Autodesk Inventor part; units mm, degrees
ref_plane "YZ Plane" through (0, 0, 0) normal (1, 0, 0) x (0, 1, 0)
ref_plane "XZ Plane" through (0, 0, 0) normal (0, 1, 0) x (-1, 0, 0)
ref_plane "XY Plane" through (0, 0, 0) normal (0, 0, 1) x (1, 0, 0)
sketch "Boceto1" plane through (0, 0, 0) normal (0, 1, 0) x (-1, 0, 0)
  line L0 (200, 200) -> (-200, 200)
  line L1 (-200, 200) -> (-200, -200)
  line L2 (-200, -200) -> (200, -200)
  line L3 (200, -200) -> (200, 200)
  point P0 (0, 0)
  dimension "d0" = 400
  dimension "L" = 400
  dimension "d2" = 200
  dimension "d3" = 200
extrude "Extrusión1" add sketch "Boceto1" along normal blind 150
sketch "Boceto3" plane through (0, 150, 0) normal (0, 1, 0) x (1, 0, 0)
  circle A0 centre (0, 160) radius 10
  line L0 (200, 200) -> (-200, 200)
  point P0 (0, 0)
  dimension "d6" = 20
  dimension "d9" = 40
extrude "Extrusión2" cut sketch "Boceto3" against normal blind 153.75
ref_plane "Plano de trabajo1" through (0, 0, 200) normal (1, 0, 0) x (0, 0, -1)
ref_plane "Plano de trabajo2" through (-200, 0, 0) normal (0, 0, 1) x (1, 0, 0)
equation "\"d0\" = L"
properties part number "CajaBoya"
Here's how the part is built. I have some questions about the finished solid (model axes, mm). Round coordinates to 2 decimals unless told otherwise and drop trailing zeros. Write each loop counter-clockwise with the first axis right and the second up, starting at its lowest first coordinate (ties: lowest second). Pieces come first, ordered by that corner, then holes.
1. I need wall thicknesses on L1, parallel to X at y = 68.5, z = -160; L2, parallel to Z at x = 0, y = 87.5. Which ranges of each line are inside material? Lowest first, please.
2. Suppose I cut it at A-A (z = -160). List the corners of the cut face in (x, y) for me.
3. Will this pin go through, and if not, where does the flat tip stop? pin 1 Ø16 at (x, z) = (0, -160) entering from +Y.
4. Suppose I cut it at B-B (x = 0). List the corners of the cut face in (y, z) for me.
5. If we mould it in two halves opening along X, with no side actions, what happens to faces 1 (the cylindrical face through (-2.17, 76.05, -150.24)), 2 (the flat face through (3, 74, -200)), 3 (the flat face through (-200, 74, -3))? For each: released by +X, released by -X, zero draft, split by the parting line, or undercut.
Answer sheet:
1. L1: x = -200 to -10, 10 to 200
1. L2: z = -200 to -170, -150 to 200
2. outline: (-200, 0) - (-10, 0) - (-10, 150) - (-200, 150) - close; (10, 0) - (200, 0) - (200, 150) - (10, 150) - close
3. pin 1: passes through
4. outline: (0, -200) - (150, -200) - (150, -170) - (0, -170) - close; (0, -150) - (150, -150) - (150, 200) - (0, 200) - close
5. face 1: undercut
5. face 2: zero draft
5. face 3: released by -X
